Autodesk Inventor part; units mm, degrees
ref_plane "YZ Plane" through (0, 0, 0) normal (1, 0, 0) x (0, 1, 0)
ref_plane "XZ Plane" through (0, 0, 0) normal (0, 1, 0) x (-1, 0, 0)
ref_plane "XY Plane" through (0, 0, 0) normal (0, 0, 1) x (1, 0, 0)
sketch "Esboço2" plane through (0, 0, 0) normal (0, 1, 0) x (-1, 0, 0)
  line L0 (-33.3088, 0) -> (-218.4, 0)
  line L1 (-218.4, 0) -> (-218.4, -20.4)
  line L2 (-218.4, -20.4) -> (-33.3088, -20.4)
  line L3 (-38.4, -19.2) -> (-218.4, -19.2)
  line L4 (-218.4, -1.2) -> (-38.4, -1.2)
  circle A0 centre (-38.4, -10.2) radius 9
  line L5 (-47.4, -20.4) -> (-47.4, -19.2)
  line L6 (-47.4, -1.2) -> (-47.4, 0)
  arc A1 (-33.3088, -20.4) -> (-33.3088, 0) centre (-38.4, -10.2) ccw
  arc A2 (-38.4, -20.4) -> (-38.4, 0) centre (-38.4, -10.2) ccw
  line L7 (-33.3088, 0) -> (0, 0)
  line L8 (0, 0) -> (0, -20.4)
  line L9 (0, -20.4) -> (-33.3088, -20.4)
  circle A3 centre (-13.5, -10.2) radius 9
  point P0 (0, -10.2)
  point P1 (-33.3088, -20.4)
  dimension "d6" = 20.4
  dimension "d8" = 1.2
  dimension "d11" = 1.2
  dimension "d25" = 18
  dimension "d44" = 1.2
  dimension "d45" = 1.2
  dimension "d46" = 180
  dimension "d47" = 27
  dimension "d48" = 18
  dimension "d49" = 13.5
extrude "Extrusão1" add sketch "Esboço2" against normal blind 1.2 contours A1 L2 A2 L0 | L7 L8 L9 A1 | A2 L2 L5 L3 A0 L4 L6 L0 | L6 L4 L1 L0 | L4 A0 L3 L1 | L2 L1 L3 L5 | A0 | A3
extrude "Extrusão2" add sketch "Esboço2" along normal blind 9 contours L7 L8 L9 A1 | A2 L2 L5 L3 A0 L4 L6 L0 | L6 L4 L1 L0 | L2 L1 L3 L5
fillet "Arredondamento6" radius 9 4 edges at (128.4, 0, -1.2) (128.4, 0, -19.2) (29.4, 0, -10.2) (22.5, 0, -10.2)
sketch "Esboço6" plane through (0, -1.2, 0) normal (0, 0, 1) x (1, 0, 0)
  line L0 (218.4, 10.2) -> (0, 10.2)
  line L1 (0, 10.2) -> (0, 6.6)
  line L2 (0, 6.6) -> (218.4, 6.6)
  line L3 (218.4, 6.6) -> (218.4, 10.2)
  line L4 (218.4, 1.2) -> (218.4, 10.2)
  line L5 (0, 10.2) -> (0, 0)
  line L6 (38.4, 10.2) -> (218.4, 10.2)
  line L7 (38.4, 1.2) -> (218.4, 1.2)
  point P0 (0, 1.2)
  point P1 (218.4, 8.4)
  point P2 (218.4, 5.7)
  point P3 (0, 8.4)
  point P4 (0, 5.1)
  point P5 (109.2, 10.2)
  point P6 (128.4, 10.2)
  dimension "d50" = 5.4
extrude "Extrusão8" cut sketch "Esboço6" against normal up to surface (20.4 mm away)
extrude "Extrusão9" add sketch "Esboço2" along normal blind 9 contours A1 L2 A2 L0
sketch "Esboço7" plane through (0, -1.2, 0) normal (0, -1, 0) x (1, 0, 0)
  line L0 (105.3, -11.4) -> (113.1, -11.4)
  line L1 (113.1, -11.4) -> (113.1, -9)
  line L2 (113.1, -9) -> (105.3, -9)
  line L3 (105.3, -9) -> (105.3, -11.4)
  line L4 (0, 0) -> (0, -20.4)
  line L5 (218.4, -20.4) -> (218.4, 0)
  arc A0 (38.4, 0) -> (38.4, -20.4) centre (38.4, -10.2) ccw
  line L6 (218.4, 0) -> (0, 0)
  point P0 (105.3, -10.2)
  point P1 (0, -10.2)
  point P2 (109.2, -9)
  point P3 (0, -10.2)
  point P4 (28.2, -10.2)
  point P5 (109.2, 0)
  dimension "d56" = 7.8
  dimension "d57" = 2.4
  dimension "d76" = 105.3
  dimension "d77" = 105.3
extrude "Extrusão10" add sketch "Esboço7" along normal blind 5.4
sketch "Esboço8" plane through (105.3, -1.2, -9) normal (0, 0, 1) x (1, 0, 0)
  circle A0 centre (3.9, -2.7) radius 1.5
  line L0 (113.1, 0) -> (-105.3, 0)
  arc A1 (1.2, -2.7) -> (6.6, -2.7) centre (3.9, -2.7) ccw
  line L1 (1.2, -2.7) -> (1.2, -1.2)
  line L2 (6.6, -2.7) -> (6.6, -1.2)
  line L3 (0, 0) -> (0, 0)
  line L4 (7.8, 0) -> (7.8, 0)
  line L5 (0, 0) -> (0, -5.4)
  line L6 (0, 0) -> (0, -5.4)
  line L7 (7.8, 0) -> (7.8, -5.4)
  line L8 (0, -5.4) -> (7.8, -5.4)
  line L9 (7.8, -5.4) -> (7.8, 0)
  arc A2 (1.2, -1.2) -> (0, 0) centre (0, -1.2) ccw
  arc A3 (7.8, 0) -> (6.6, -1.2) centre (7.8, -1.2) ccw
  point P0 (-105.3, 1.2)
  point P1 (3.9, 0)
  point P2 (1.2, 0)
  point P3 (6.6, 0)
  point P4 (1.2, 0)
  point P5 (6.6, 0)
  point P6 (0, 0)
  point P7 (3.9, 0)
  point P8 (7.8, 0)
  point P9 (3.9, -5.4)
  point P10 (3.9, -5.4)
  dimension "d61" = 3
  dimension "d62" = 2.7
  dimension "d65" = 1.2
  dimension "d66" = 1.2
extrude "Extrusão11" cut sketch "Esboço8" against normal up to surface (2.4 mm away) contours A0 | L7 L8 A1 L2 A3 | A2 L1 A1 L8 L5
equation "\"d6\" = Diâmetro_esfera + 2 * Margem"
equation "\"d8\" = Margem"
equation "\"d11\" = Margem"
equation "\"d25\" = Diâmetro_esfera"
equation "\"d44\" = Margem"
equation "\"d45\" = Margem"
equation "\"d46\" = 10 * Diâmetro_esfera"
equation "\"d48\" = Diâmetro_esfera"
equation "\"d49\" = 0.5 * d47"
equation "\"d13\" = Margem"
equation "\"d15\" = 0.5 * Diâmetro_esfera"
equation "\"d55\" = 0.5 * Diâmetro_esfera"
equation "\"d50\" = 0.3 * Diâmetro_esfera"
equation "\"d53\" = 0.5 * Diâmetro_esfera"
equation "\"d56\" = Parafuso + 4 * Margem"
equation "\"d57\" = 2 * Margem"
equation "\"d59\" = Parafuso + 2 * Margem"
equation "\"d61\" = Parafuso"
equation "\"d62\" = 0.5 * Parafuso + Margem"
equation "\"d65\" = Margem"
equation "\"d67\" = Parafuso + 2 * Margem"
equation "\"Diâmetro_esfera\" = 18"
equation "\"Margem\" = 3 * Filamento"
equation "\"Filamento\" = 0.4"
equation "\"Parafuso\" = 3"
equation "\"d42\" = Margem"
equation "\"d43\" = Margem"
equation "\"Tamanho_receptor\" = 37.257"
properties part number "Trilho 60 minutos  - 12 horas" material "Plástico PET"
The listing builds one solid part. Answer for the finished solid, in the listing's coordinates (mm). A direction names the side the tool comes from. Coordinates: 2 decimals unless noted, no trailing zeros.
Q1. Consider line 1 (Y direction, x = 109.2, z = -10.3); line 2 (Y direction, x = 43, z = -1.5); line 3 (Y direction, x = 108.5, z = -9.5). Determine where each line is inside the solid, lowest interval first.
Q2. For a pull along Z with two mould halves and no side action, classify faces 6 (the face through (28, 9, -10)), 7 (the face through (109, -2, -9)), 8 (the face through (28.2, 7.2, -10)) as pulls with the +Z half, pulls with the -Z half, needs draft (parallel to the pull), parting line crosses it, or undercut.
Q3. Given P1, Ø4, axis at x = 71.5, y = 0, coming from the +Z side; P2, Ø8, axis at x = 62.5, z = -5, coming from the -Y side; P3, Ø6, axis at x = 165, z = -13, coming from the +Y side; P4, Ø0.8, axis at y = -3, z = -9.5, coming from the +X side, each flat-ended and moving along its own axis, determine where each tip first touches the part or whether it passes through.
Q4. Which of the six approach directions +Z, -Z, +X, -X, +Y, -Y give full straight-line access (tool end or side, diameter ignored) to faces 1 (the face through (27, 7, -10)), 2 (the face through (109, -2, -11.4)), 3 (the face through (129.66, 1.51, -5.21)), 4 (the face through (0, 2, -10)), 5 (the face through (218.4, -1, -10))?
Answers follow:
1. line 1: y = -6.6 to -5.4, -2.4 to 0
1. line 2: y = -1.2 to 5.4
1. line 3: y = -6.51 to -5.23, -2.57 to 0.03
2. face 6: needs draft
2. face 7: pulls with the +Z half
2. face 8: undercut
3. P1: stops at z = 0
3. P2: stops at y = -1.2
3. P3: stops at y = 2.12
3. P4: stops at x = 111.9
4. face 1: -X, +Y
4. face 2: -Z, +X, -X, -Y
4. face 3: +X, +Y
4. face 4: +Z, -Z, -X, +Y, -Y
4. face 5: +Z, -Z, +X, +Y, -Y
